Source: CAD feature listing. Evaluate the final solid. Frame: model axes, mm. A direction names the side the tool comes from. Give positions to 0.01 mm unless a question says otherwise; leave off trailing zeros. Write each loop counter-clockwise with the first axis right and the second up, starting at its lowest first coordinate (ties: lowest second). Pieces come first, ordered by that corner, then holes. Notation, with made-up numbers: (85, 9.5) -> (113, 9.5) arc R14 cw to (113, 13.5) -> close; hole circle Ø9 at (-23, 86). An arc over 180 degrees is marked (long way). Use a Markdown table: item, result. Add a question column.
```python
from build123d import *

# Parameters (mm, degrees)
SKETCH2_W               = 28.77498914
SKETCH2_H               = 18
SKETCH2_R               = 2
BOSS_EXTRUDE1_DEPTH     = 6.37
CUT_EXTRUDE1_REACH      = 11.63
SKETCH3_W               = 27.288002312
SKETCH3_H               = 18
CUT_EXTRUDE2_START      = -14.387495
SKETCH2_2_W             = 28.77498914
SKETCH2_2_H             = 18
SKETCH2_2_R             = 2
CUT_EXTRUDE2_DEPTH      = 8.017495
FILLET1_R               = 6
CUT_EXTRUDE3_DEPTH      = 17
CUT_EXTRUDE3_DEPTH_BACK = 17


with BuildPart() as part:
    # Sketch1 → Revolve1 (revolve)
    with BuildSketch(Plane.XY):
        with BuildLine():
            Line((0, 16), (0, -16))
            ThreePointArc((0, -16), (16, 0), (0, 16))
        make_face()
    revolve(axis=Axis((0, 16, 0), (0, -1, 0)))

    # Sketch2 → Boss-Extrude1 (add, symmetric)
    with BuildSketch(Plane.XY):
        with Locations((0, 16)):
            Rectangle(SKETCH2_W, SKETCH2_H)
        with Locations((-6, 19)):
            Circle(SKETCH2_R, mode=Mode.SUBTRACT)
        with Locations((6, 19)):
            Circle(SKETCH2_R, mode=Mode.SUBTRACT)
        Polygon((0, 16.599186911), (-3.55, 14.549593456), (-3.55, 10.450406544), (0, 8.400813089), (3.55, 10.450406544), (3.55, 14.549593456), align=None, mode=Mode.SUBTRACT)
    extrude(amount=BOSS_EXTRUDE1_DEPTH, both=True)

    # Sketch3 → Cut-Extrude1 (cut, up to next)
    with BuildSketch(Plane.XY.offset(6.37), mode=Mode.PRIVATE) as cut_extrude1_sk1:
        with Locations((-0.743493414, 16)):
            Rectangle(SKETCH3_W, SKETCH3_H)
    cut_extrude1_tool1 = extrude(cut_extrude1_sk1.sketch, amount=CUT_EXTRUDE1_REACH, mode=Mode.PRIVATE) & part.part
    add(cut_extrude1_tool1.solids().sort_by_distance((-0.743493, 16, 6.37))[0], mode=Mode.SUBTRACT)

    # Sketch2<2> → Cut-Extrude2 (cut)
    with BuildSketch(Plane.XY.offset(CUT_EXTRUDE2_START)):
        Polygon((3.55, 10.450406544), (3.55, 14.549593456), (0, 16.599186911), (-3.55, 14.549593456), (-3.55, 10.450406544), (0, 8.400813089), align=None)
        with Locations((0, 16)):
            Rectangle(SKETCH2_2_W, SKETCH2_2_H)
        with Locations((6, 19)):
            Circle(SKETCH2_2_R, mode=Mode.SUBTRACT)
        with Locations((-6, 19)):
            Circle(SKETCH2_2_R, mode=Mode.SUBTRACT)
        Polygon((3.55, 14.549593456), (0, 16.599186911), (-3.55, 14.549593456), (-3.55, 10.450406544), (0, 8.400813089), (3.55, 10.450406544), align=None, mode=Mode.SUBTRACT)
    extrude(amount=CUT_EXTRUDE2_DEPTH, mode=Mode.SUBTRACT)

    # Fillet1
    fillet1_edges = [part.edges().sort_by_distance(p)[0] for p in [
        (-14.38749457, 25, 0),
        (14.38749457, 25, 0),
    ]]
    fillet(fillet1_edges, radius=FILLET1_R)

    # Sketch2<3> → Cut-Extrude3 (cut, two sides)
    with BuildSketch(Plane.XY) as cut_extrude3_sk:
        Polygon((0, 16.599186911), (-3.55, 14.549593456), (-3.55, 10.450406544), (0, 8.400813089), (3.55, 10.450406544), (3.55, 14.549593456), align=None)
    extrude(amount=CUT_EXTRUDE3_DEPTH, mode=Mode.SUBTRACT)
    extrude(cut_extrude3_sk.sketch, amount=-CUT_EXTRUDE3_DEPTH_BACK, mode=Mode.SUBTRACT)


solid = part.part
```
(1) Mould query, pull axis Y, two halves, no side actions, for faces 6 (the flat face through (14.387, 13, 0)), 7 (the cylindrical face through (12.58, 23.29, -0.09)), 8 (the flat face through (3.55, 12, 0)). Classes: +Y half, -Y half, draft (parallel to the pull), parting line (faces both ways), or undercut.
(2) Cut plane B-B on x = 6. Return the cut outline in (y, z), then the cut area to 3 significant figures.
(3) Material intervals for L1, parallel to Y at x = -6, z = 3; L2, parallel to Y at x = -6, z = -2; L3, parallel to Z at x = -3, y = 17, sorted ascending.
(4) First-contact query: pin 1 Ø14.5 at (x, y) = (-4.5, 19.5) entering from -Z; pin 2 Ø4.5 at (y, z) = (13, -2) entering from -X; pin 3 Ø12 at (x, y) = (-9, -2.5) entering from -Z; pin 4 Ø4 at (x, z) = (-0.5, 7) entering from +Y. Flat tips, straight axial feed; report the tip coordinate or a pass-through.
(5) Access query for faces 1 (the flat face through (0, 7, -10)), 2 (the cylindrical face through (-12.677, 23.196, -0.089)), 3 (the flat face through (0, 25, 0)), 4 (the flat face through (0, 18, 6.37)), 5 (the flat face through (-3.55, 13, 0)). Directions: +Z, -Z, +X, -X, +Y, -Y. A direction counts if a zero-diameter tool reaches every point of the face in a straight line with its end or side. Return the directions, or none.
(6) Cut plane D-D on y = 2. Return the cut outline in (x, z), then the cut area to 3 significant figures.
(7) Cut plane A-A on z = -4. Return the cut outline in (x, y).
(8) Cut plane C-C on y = -10.5. Return the cut outline in (x, z), then the cut area to 3 significant figures.
Output:
| question | item | result |
|---|---|---|
| 1 | face 6 | draft |
| 1 | face 7 | +Y half |
| 1 | face 8 | undercut |
| 2 | outline | (7, -13.08) -> (7, -6.37) -> (17, -6.37) -> (17, 6.37) -> (7, 6.37) -> (7, 13.08) arc R14.83 ccw (long way) to start; (21, -6.37) -> (25, -6.37) -> (25, 6.37) -> (21, 6.37) -> close |
| 2 | area | 724 mm^2 |
| 3 | L1 | -14.53 to 17, 21 to 25 |
| 3 | L2 | -14.7 to 17, 21 to 25 |
| 3 | L3 | -6.37 to 6.37 |
| 4 | pin 1 | z = -6.37 |
| 4 | pin 2 | x = -14.39 |
| 4 | pin 3 | z = -15.65 |
| 4 | pin 4 | y = 25 |
| 5 | face 1 | -Z, +X, -X, +Y |
| 5 | face 2 | +Z, -Z, -X, +Y |
| 5 | face 3 | +Z, -Z, +X, -X, +Y |
| 5 | face 4 | +Z, +X, -X, +Y |
| 5 | face 5 | +Z, -Z |
| 6 | outline | circle Ø31.75 at (0, 0) |
| 6 | area | 792 mm^2 |
| 7 | outline | (-14.39, 7) -> (-13.82, 7) arc R15.49 ccw (long way) to (13.82, 7) -> (14.39, 7) -> (14.39, 19) arc R6 ccw to (8.39, 25) -> (-8.39, 25) arc R6 ccw to (-14.39, 19) -> close; hole circle Ø4 at (-6, 19); hole (-3.55, 10.45) -> (0, 8.4) -> (3.55, 10.45) -> (3.55, 14.55) -> (0, 16.6) -> (-3.55, 14.55) -> close; hole circle Ø4 at (6, 19) |
| 8 | outline | circle Ø24.15 at (0, 0) |
| 8 | area | 458 mm^2 |
